Could you check a few things on this model? Use its own coordinates, in mm. Round coordinates to 2 decimals unless told otherwise and drop trailing zeros. Order: outer loops, then holes, each group sorted by start corner. A loop starts at its lowest first (then second) coordinate and runs counter-clockwise, first axis right, second up. Notation, with made-up numbers: (87.5, -38) -> (137.5, -38) arc R17 cw to (137.5, -14) -> close; hole circle Ø6 at (-35.75, 74.5). An arc over 180 degrees is marked (long way). One line per question, with ' | ' between items.
```python
from build123d import *

# Parameters (mm, degrees)
BOSS_EXTRU_1_OUTLINE_R   = 50
BOSS_EXTRU_1_OUTLINE_W   = 5
BOSS_EXTRU_1_OUTLINE_H   = 5
BOSS_EXTRU_1_OUTLINE_R_2 = 2.05
BOSS_EXTRU_1_OUTLINE_R_3 = 1.5
BOSS_EXTRU_1_DEPTH       = 5
SKETCH3_W                = 1
SKETCH3_H                = 8
CUT_EXTRUDE2_DEPTH       = 10
SKETCH4_R                = 7.5
CUT_EXTRUDE3_DEPTH       = 10


# Read off the part's stored shape, not the designer's step: Boss.-Extru.1
with BuildPart() as part:
    # Boss.-Extru.1 outline → Boss.-Extru.1 (new body)
    with BuildSketch(Plane.XY):
        Circle(BOSS_EXTRU_1_OUTLINE_R)
        Polygon((-37.262039705, -33.060254038), (-39.762039705, -28.730127019), (-35.431912686, -26.230127019), (-32.931912686, -30.560254038), align=None, mode=Mode.SUBTRACT)
        with Locations((-7.5, -46.3)):
            Rectangle(BOSS_EXTRU_1_OUTLINE_W, BOSS_EXTRU_1_OUTLINE_H, mode=Mode.SUBTRACT)
        with Locations((-16.666666667, -28.867513459)):
            Circle(BOSS_EXTRU_1_OUTLINE_R_2, mode=Mode.SUBTRACT)
        with Locations((-40.096976195, -23.15)):
            Circle(BOSS_EXTRU_1_OUTLINE_R_3, mode=Mode.SUBTRACT)
        Polygon((-42.931912686, -13.239745962), (-40.431912686, -17.569872981), (-44.762039705, -20.069872981), (-47.262039705, -15.739745962), align=None, mode=Mode.SUBTRACT)
        with Locations((-34.597845014, -19.975075132)):
            Circle(BOSS_EXTRU_1_OUTLINE_R_2, mode=Mode.SUBTRACT)
        with Locations((-16.671397033, -9.625235564)):
            Circle(BOSS_EXTRU_1_OUTLINE_R_2, mode=Mode.SUBTRACT)
        with Locations((0, -46.3)):
            Circle(BOSS_EXTRU_1_OUTLINE_R_3, mode=Mode.SUBTRACT)
        with Locations((7.5, -46.3)):
            Rectangle(BOSS_EXTRU_1_OUTLINE_W, BOSS_EXTRU_1_OUTLINE_H, mode=Mode.SUBTRACT)
        with Locations((0, -39.950150265)):
            Circle(BOSS_EXTRU_1_OUTLINE_R_2, mode=Mode.SUBTRACT)
        with Locations((16.666666667, -28.867513459)):
            Circle(BOSS_EXTRU_1_OUTLINE_R_2, mode=Mode.SUBTRACT)
        Polygon((32.931912686, -30.560254038), (35.431912686, -26.230127019), (39.762039705, -28.730127019), (37.262039705, -33.060254038), align=None, mode=Mode.SUBTRACT)
        with Locations((0, -19.232757636)):
            Circle(BOSS_EXTRU_1_OUTLINE_R_2, mode=Mode.SUBTRACT)
        with Locations((16.666666667, -9.622504487)):
            Circle(BOSS_EXTRU_1_OUTLINE_R_2, mode=Mode.SUBTRACT)
        with Locations((34.597845014, -19.975075132)):
            Circle(BOSS_EXTRU_1_OUTLINE_R_2, mode=Mode.SUBTRACT)
        with Locations((40.096976195, -23.15)):
            Circle(BOSS_EXTRU_1_OUTLINE_R_3, mode=Mode.SUBTRACT)
        Polygon((47.262039705, -15.739745962), (44.762039705, -20.069872981), (40.431912686, -17.569872981), (42.931912686, -13.239745962), align=None, mode=Mode.SUBTRACT)
        with Locations((-33.333333333, 0)):
            Circle(BOSS_EXTRU_1_OUTLINE_R_2, mode=Mode.SUBTRACT)
        Polygon((-47.262039705, 15.739745962), (-44.762039705, 20.069872981), (-40.431912686, 17.569872981), (-42.931912686, 13.239745962), align=None, mode=Mode.SUBTRACT)
        with Locations((-40.096976195, 23.15)):
            Circle(BOSS_EXTRU_1_OUTLINE_R_3, mode=Mode.SUBTRACT)
        with Locations((-34.597845014, 19.975075132)):
            Circle(BOSS_EXTRU_1_OUTLINE_R_2, mode=Mode.SUBTRACT)
        with Locations((-16.671397032, 9.625235564)):
            Circle(BOSS_EXTRU_1_OUTLINE_R_2, mode=Mode.SUBTRACT)
        Polygon((-32.931912686, 30.560254038), (-35.431912686, 26.230127019), (-39.762039705, 28.730127019), (-37.262039705, 33.060254038), align=None, mode=Mode.SUBTRACT)
        with Locations((-16.666666667, 28.867513459)):
            Circle(BOSS_EXTRU_1_OUTLINE_R_2, mode=Mode.SUBTRACT)
        with Locations((-7.5, 46.3)):
            Rectangle(BOSS_EXTRU_1_OUTLINE_W, BOSS_EXTRU_1_OUTLINE_H, mode=Mode.SUBTRACT)
        Circle(BOSS_EXTRU_1_OUTLINE_R_2, mode=Mode.SUBTRACT)
        with Locations((16.669571796, 9.624181764)):
            Circle(BOSS_EXTRU_1_OUTLINE_R_2, mode=Mode.SUBTRACT)
        with Locations((0, 19.165334425)):
            Circle(BOSS_EXTRU_1_OUTLINE_R_2, mode=Mode.SUBTRACT)
        with Locations((33.333333333, 0)):
            Circle(BOSS_EXTRU_1_OUTLINE_R_2, mode=Mode.SUBTRACT)
        with Locations((34.597845014, 19.975075133)):
            Circle(BOSS_EXTRU_1_OUTLINE_R_2, mode=Mode.SUBTRACT)
        Polygon((42.931912686, 13.239745962), (40.431912686, 17.569872981), (44.762039705, 20.069872981), (47.262039705, 15.739745962), align=None, mode=Mode.SUBTRACT)
        with Locations((40.096976195, 23.15)):
            Circle(BOSS_EXTRU_1_OUTLINE_R_3, mode=Mode.SUBTRACT)
        with Locations((16.666666667, 28.867513459)):
            Circle(BOSS_EXTRU_1_OUTLINE_R_2, mode=Mode.SUBTRACT)
        with Locations((0, 39.950150265)):
            Circle(BOSS_EXTRU_1_OUTLINE_R_2, mode=Mode.SUBTRACT)
        with Locations((0, 46.3)):
            Circle(BOSS_EXTRU_1_OUTLINE_R_3, mode=Mode.SUBTRACT)
        with Locations((7.5, 46.3)):
            Rectangle(BOSS_EXTRU_1_OUTLINE_W, BOSS_EXTRU_1_OUTLINE_H, mode=Mode.SUBTRACT)
        Polygon((37.262039705, 33.060254038), (39.762039705, 28.730127019), (35.431912686, 26.230127019), (32.931912686, 30.560254038), align=None, mode=Mode.SUBTRACT)
    extrude(amount=BOSS_EXTRU_1_DEPTH)

    # Sketch3 → Cut-Extrude2 (cut)
    with BuildSketch(Plane.XY.offset(5)):
        with Locations((-22.833333333, 0)):
            Rectangle(SKETCH3_W, SKETCH3_H)
        Polygon((-13.233653965, 23.921361037), (-14.099679369, 23.421361037), (-12.349679369, 20.390272124), (-15.380768282, 18.640272124), (-14.880768282, 17.77424672), (-11.849679369, 19.52424672), (-10.099679369, 16.493157806), (-9.233653965, 16.993157806), (-10.983653965, 20.02424672), (-7.952565052, 21.77424672), (-8.452565052, 22.640272124), (-11.483653965, 20.890272124), align=None)
        Polygon((15.311458483, 17.894294813), (14.811458483, 17.028269409), (7.883255253, 21.028269409), (8.383255253, 21.894294813), align=None)
        Polygon((8.02187485, -22.52022403), (7.52187485, -21.654198627), (14.450078081, -17.654198627), (14.950078081, -18.52022403), align=None)
        Polygon((27.333333333, -0.5), (27.333333333, 0.5), (23.833333333, 0.5), (23.833333333, 4), (22.833333333, 4), (22.833333333, 0.5), (19.333333333, 0.5), (19.333333333, -0.5), (22.833333333, -0.5), (22.833333333, -4), (23.833333333, -4), (23.833333333, -0.5), align=None)
        Polygon((-14.099679369, -23.421361037), (-13.233653965, -23.921361037), (-11.483653965, -20.890272124), (-8.452565052, -22.640272124), (-7.952565052, -21.77424672), (-10.983653965, -20.02424672), (-9.233653965, -16.993157806), (-10.099679369, -16.493157806), (-11.849679369, -19.52424672), (-14.880768282, -17.77424672), (-15.380768282, -18.640272124), (-12.349679369, -20.390272124), align=None)
        Polygon((-7.005935602, -0.708643072), (-7.005935602, 0.291356928), (-10.505935602, 0.291356928), (-10.505935602, 3.791356928), (-11.505935602, 3.791356928), (-11.505935602, 0.291356928), (-15.005935602, 0.291356928), (-15.005935602, -0.708643072), (-11.505935602, -0.708643072), (-11.505935602, -4.208643072), (-10.505935602, -4.208643072), (-10.505935602, -0.708643072), align=None)
        Polygon((-24.636137397, -11.902985286), (-23.7450767, -13.444692017), (-24.087572192, -13.64217549), (-24.97863289, -12.100468759), align=None)
    extrude(amount=-CUT_EXTRUDE2_DEPTH, mode=Mode.SUBTRACT)

    # Sketch4 → Cut-Extrude3 (cut)
    with BuildSketch(Plane(origin=(0, 0, 0), x_dir=(-1, 0, 0), z_dir=(0, 0, -1))):
        with Locations((-33.333333333, 0)):
            Circle(SKETCH4_R)
        Circle(SKETCH4_R)
        with Locations((33.333333333, 0)):
            Circle(SKETCH4_R)
        with Locations((16.671397033, -9.625235564)):
            Circle(SKETCH4_R)
        with BuildLine():
            Line((16.666666667, -36.367513459), (-16.666666667, -36.367513459))
            ThreePointArc((-16.666666667, -36.367513459), (-24.166666667, -28.867513459), (-16.666666667, -21.367513459))
            Line((-16.666666667, -21.367513459), (16.666666667, -21.367513459))
            ThreePointArc((16.666666667, -21.367513459), (24.166666667, -28.867513459), (16.666666667, -36.367513459))
        make_face()
        with BuildLine():
            Line((-16.666666667, 36.367513459), (16.666666667, 36.367513459))
            ThreePointArc((16.666666667, 36.367513459), (24.166666667, 28.867513459), (16.666666667, 21.367513459))
            Line((16.666666667, 21.367513459), (-16.666666667, 21.367513459))
            ThreePointArc((-16.666666667, 21.367513459), (-24.166666667, 28.867513459), (-16.666666667, 36.367513459))
        make_face()
    extrude(amount=-CUT_EXTRUDE3_DEPTH, mode=Mode.SUBTRACT)


with BuildPart() as cut_extrude3_kept_piece:
    # of the separate pieces the step leaves, the one the design keeps (cut_extrude3_pieces_kept)
    add(part.part.solids().sort_by_distance((50, 0, 0))[0])


solid = cut_extrude3_kept_piece.part
```
1. I need wall thicknesses on probe 1 along X at (y, z) = (6, 2.5); probe 2 along X at (y, z) = (27, 3.7); probe 3 along Y at (x, z) = (-8, 3.75). Which ranges of each line are inside material? Lowest first, please.
From the geometry:
probe 1: x = -49.64 to -37.83, -28.83 to -4.5, 4.5 to 28.83, 37.83 to 49.64 | probe 2: x = -42.08 to -36.77, -34.99 to -23.93, 23.93 to 34.99, 36.77 to 42.08 | probe 3: y = -49.36 to -48.8, -43.8 to -36.37, -21.37 to -0.71, 0.29 to 21.37, 36.37 to 43.8, 48.8 to 49.36
2. I want a section at B-B on y = -46.3. List the corners of the cut face in (x, z) for me, and give its area (3 significant figures).
From the geometry:
outline: (-18.88, 0) -> (-10, 0) -> (-10, 5) -> (-18.88, 5) -> close; (-5, 0) -> (-1.5, 0) -> (-1.5, 5) -> (-5, 5) -> close; (1.5, 0) -> (5, 0) -> (5, 5) -> (1.5, 5) -> close; (10, 0) -> (18.88, 0) -> (18.88, 5) -> (10, 5) -> close | area: 124 mm²
3. I want a section at C-C on x = -27. List the corners of the cut face in (y, z) for me, and give its area (3 significant figures).
From the geometry:
outline: (-42.08, 0) -> (-4.02, 0) -> (-4.02, 5) -> (-42.08, 5) -> close; (4.02, 0) -> (42.08, 0) -> (42.08, 5) -> (4.02, 5) -> close | area: 381 mm²
4. I'm going to push flat-ended pins straight in: pin 1 (3 mm diameter, centred on y = -36, z = 2, fed in from +X); pin 2 (2.5 mm diameter, centred on y = -45.5, z = 2, fed in from +X); pin 3 (1.1 mm diameter, centred on x = 23, z = 2.5, fed in from -Y); pin 4 (2.5 mm diameter, centred on x = -16.67, y = 9.63, fed in from +Z). Where does each tip first touch, or does it pass through?
From the geometry:
pin 1: stops at x = 36.19 | pin 2: stops at x = 23.28 | pin 3: stops at y = -44.68 | pin 4: passes through
5. If we mould it in two halves opening along Y, with no side actions, what happens to faces 1 (the face through (10, 1, 0)), 2 (the face through (40.826, 0.323, 2.465))? For each: pulls with the +Y half, pulls with the -Y half, needs draft (parallel to the pull), parting line crosses it, or undercut.
From the geometry:
face 1: needs draft | face 2: undercut
6. I want a section at A-A on x = 0. Count the separate pieces of the cut face and the enclosed holes in it, and give its area (3 significant figures).
From the geometry:
separate pieces: 10 | enclosed holes: 0 | area: 163 mm²
